Work out the finished part from the listing and answer in its coordinate system (mm). A direction names the side the tool comes from. Coordinates: 2 decimals unless noted, no trailing zeros. Order: outer loops, then holes, each group sorted by start corner. A loop starts at its lowest first (then second) coordinate and runs counter-clockwise, first axis right, second up.
```python
from build123d import *

# Parameters (mm, degrees)
SKETCH058_W          = 85
SKETCH058_H          = 10
SKETCH058_R          = 1.6
PAD030_DEPTH         = 10
FILLET019_R          = 3
SKETCH059_W          = 80
SKETCH059_H          = 5
PAD031_DEPTH         = 10
SKETCH060_W          = 61
SKETCH060_H          = 3.5
POCKET027_DEPTH      = 10.001
FILLET020_R          = 4
CHAMFER014_SIZE      = 5
SKETCH061_R          = 1.6
POCKET028_DEPTH      = 10.001
POCKET028_DEPTH_BACK = 5.001
CHAMFER015_SIZE      = 1.9
SKETCH062_R          = 2.3
POCKET029_DEPTH      = 7
CHAMFER016_SIZE      = 1
FILLET021_R          = 10
FILLET022_R          = 3
CHAMFER017_SIZE      = 0.5
SKETCH063_R          = 3.5
POCKET030_DEPTH      = 3
SKETCH064_R          = 3.5
POCKET031_DEPTH      = 3
SKETCH065_W          = 72
SKETCH065_H          = 3.5
POCKET032_DEPTH      = 10.001
FILLET023_R          = 2
FILLET024_R          = 5
CHAMFER018_SIZE      = 1
CHAMFER019_SIZE      = 1
CHAMFER020_SIZE      = 0.4


with BuildPart() as part:
    # Sketch058 → Pad030 (new body)
    with BuildSketch(Plane.XY):
        with Locations((-37.5, 0)):
            Rectangle(SKETCH058_W, SKETCH058_H)
        Circle(SKETCH058_R, mode=Mode.SUBTRACT)
    extrude(amount=PAD030_DEPTH)

    # Fillet019
    fillet019_edges = [part.edges().sort_by_distance(p)[0] for p in [
        (5, 5, 5),
        (5, -5, 5),
    ]]
    fillet(fillet019_edges, radius=FILLET019_R)

    # Sketch059 → Pad031 (join)
    with BuildSketch(Plane.XY):
        with Locations((-40, 7.5)):
            Rectangle(SKETCH059_W, SKETCH059_H)
    extrude(amount=PAD031_DEPTH)

    # Sketch060 → Pocket027 (cut, through all)
    with BuildSketch(Plane.XY):
        with Locations((-46.5, 6.25)):
            Rectangle(SKETCH060_W, SKETCH060_H)
    extrude(amount=POCKET027_DEPTH, mode=Mode.SUBTRACT)

    # Fillet020
    fillet020_edges = [part.edges().sort_by_distance(p)[0] for p in [
        (0, 10, 5),
        (-80, 10, 5),
    ]]
    fillet(fillet020_edges, radius=FILLET020_R)

    # Chamfer014
    chamfer014_edges = [part.edges().sort_by_distance(p)[0] for p in [
        (-80, -5, 5),
    ]]
    chamfer(chamfer014_edges, length=CHAMFER014_SIZE)

    # Sketch061 → Pocket028 (cut, two sides)
    with BuildSketch(Plane.XZ) as pocket028_sk:
        with Locations((-23, 5)):
            Circle(SKETCH061_R)
        with Locations((-70, 5)):
            Circle(SKETCH061_R)
    extrude(amount=-POCKET028_DEPTH, mode=Mode.SUBTRACT)
    extrude(pocket028_sk.sketch, amount=POCKET028_DEPTH_BACK, mode=Mode.SUBTRACT)

    # Chamfer015
    chamfer015_edges = [part.edges().sort_by_distance(p)[0] for p in [
        (-71.6, 10, 5),
        (-24.6, 10, 5),
    ]]
    chamfer(chamfer015_edges, length=CHAMFER015_SIZE)

    # Sketch062 (on Face11 of Chamfer015) → Pocket029 (cut)
    with BuildSketch(Plane.XZ.offset(5)):
        with Locations((-70, 5)):
            Circle(SKETCH062_R)
        with Locations((-23, 5)):
            Circle(SKETCH062_R)
    extrude(amount=-POCKET029_DEPTH, mode=Mode.SUBTRACT)

    # Chamfer016
    chamfer016_edges = [part.edges().sort_by_distance(p)[0] for p in [
        (-72.3, -5, 5),
        (-25.3, -5, 5),
    ]]
    chamfer(chamfer016_edges, length=CHAMFER016_SIZE)

    # Fillet021
    fillet021_edges = [part.edges().sort_by_distance(p)[0] for p in [
        (-80, 0, 5),
    ]]
    fillet(fillet021_edges, radius=FILLET021_R)

    # Fillet022
    fillet022_edges = [part.edges().sort_by_distance(p)[0] for p in [
        (-75, -5, 5),
    ]]
    fillet(fillet022_edges, radius=FILLET022_R)

    # Chamfer017
    chamfer017_edges = [part.edges().sort_by_distance(p)[0] for p in [
        (-71.6, 4.5, 5),
        (-24.6, 4.5, 5),
    ]]
    chamfer(chamfer017_edges, length=CHAMFER017_SIZE)

    # Sketch063 (on Face6 of Chamfer017) → Pocket030 (cut)
    with BuildSketch(Plane.XY.offset(10)):
        Circle(SKETCH063_R)
    extrude(amount=-POCKET030_DEPTH, mode=Mode.SUBTRACT)

    # Sketch064 (on Face3 of Pocket030) → Pocket031 (cut)
    with BuildSketch(Plane(origin=(0, 0, 0), x_dir=(1, 0, 0), z_dir=(0, 0, -1))):
        Circle(SKETCH064_R)
    extrude(amount=-POCKET031_DEPTH, mode=Mode.SUBTRACT)

    # Sketch065 → Pocket032 (cut, through all)
    with BuildSketch(Plane.XY):
        with Locations((-44, -3.25)):
            Rectangle(SKETCH065_W, SKETCH065_H)
    extrude(amount=POCKET032_DEPTH, mode=Mode.SUBTRACT)

    # Fillet023
    fillet023_edges = [part.edges().sort_by_distance(p)[0] for p in [
        (-8, -5, 5),
    ]]
    fillet(fillet023_edges, radius=FILLET023_R)

    # Fillet024
    fillet024_edges = [part.edges().sort_by_distance(p)[0] for p in [
        (-78.256289, -1.5, 5),
    ]]
    fillet(fillet024_edges, radius=FILLET024_R)

    # Chamfer018
    chamfer018_edges = [part.edges().sort_by_distance(p)[0] for p in [
        (-8, -1.5, 5),
    ]]
    chamfer(chamfer018_edges, length=CHAMFER018_SIZE)

    # Chamfer019
    chamfer019_edges = [part.edges().sort_by_distance(p)[0] for p in [
        (-72.3, -1.5, 5),
        (-25.3, -1.5, 5),
    ]]
    chamfer(chamfer019_edges, length=CHAMFER019_SIZE)

    # Chamfer020
    chamfer020_edges = [part.edges().sort_by_distance(p)[0] for p in [
        (-41.979297, -1.5, 10),
        (-8.5, -2, 10),
        (-78.259301, -0.255708, 10),
        (-8, -2.75, 10),
        (-79.979276, 3.498666, 10),
        (-7.414214, -4.414214, 10),
        (-80, 5.071068, 10),
        (-2, -5, 10),
        (-78.828427, 8.828427, 10),
        (4.12132, -4.12132, 10),
        (-40, 10, 10),
        (5, 0, 10),
        (-1.171573, 8.828427, 10),
        (4.12132, 4.12132, 10),
        (0, 5.5, 10),
        (1, 5, 10),
        (-3.5, 0, 10),
        (-46.5, 8, 10),
        (-16, 6.25, 10),
        (-77, 6.25, 10),
        (-46.5, 4.5, 10),
        (-41.979297, -1.5, 0),
        (-8.5, -2, 0),
        (-78.259301, -0.255708, 0),
        (-8, -2.75, 0),
        (-79.979276, 3.498666, 0),
        (-7.414214, -4.414214, 0),
        (-80, 5.071068, 0),
        (-2, -5, 0),
        (-78.828427, 8.828427, 0),
        (4.12132, -4.12132, 0),
        (-40, 10, 0),
        (5, 0, 0),
        (-1.171573, 8.828427, 0),
        (4.12132, 4.12132, 0),
        (0, 5.5, 0),
        (1, 5, 0),
        (-3.5, 0, 0),
        (-46.5, 8, 0),
        (-77, 6.25, 0),
        (-16, 6.25, 0),
        (-46.5, 4.5, 0),
    ]]
    chamfer(chamfer020_edges, length=CHAMFER020_SIZE)


solid = part.part
```
1. Flat-ended cylindrical pins translate along their axes: pin 1 (0.6 mm diameter, centred on y = -2.5, z = 3, fed in from -X); pin 2 (5 mm diameter, centred on x = -23, z = 5, fed in from -Y); pin 3 (1 mm diameter, centred on x = -48.5, z = 3, fed in from -Y). Find the tip coordinate at first contact, or state that the pin passes through.
2. The mould has two halves that part along Z. Classify faces 3 (the cylindrical face through (-22.26, 2.99, 3.58)), 4 (the cylindrical face through (-7.4, -4.43, 5.06)), 5 (the flat face through (-38, 3, 0)), 6 (the flat face through (-8.37, -1.85, 9.8)): released by +Z, released by -Z, zero draft, split by the parting line, or undercut.
3. The part is cut by section A-A (x = -70). Count the separate pieces of the cut face and the enclosed holes in it, plus the area to 3 significant figures.
4. The part is cut by section B-B (x = -32.5). Determine the outline of the cut face in (y, z), plus the area to 3 significant figures.
5. Consider probe 1 along Y at (x, z) = (-59.5, 9.25); probe 2 along X at (y, z) = (3.25, 3.75); probe 3 along X at (y, z) = (3.5, 6.25). Determine where each line is inside the solid, lowest interval first.
6. For faces 1 (the flat face through (-16, 6, 5)), 2 (the cylindrical face through (4.1, -4.14, 5.06)), determine the directions among +Z, -Z, +X, -X, +Y, -Y from which every point of the face is accessible in a straight line to the end or side of a thin tool.
Worked out:
1. pin 1: stops at x = -8.3
1. pin 2: stops at y = -0.7
1. pin 3: stops at y = -1.5
2. face 3: undercut
2. face 4: zero draft
2. face 5: released by -Z
2. face 6: released by +Z
3. separate pieces: 4
3. enclosed holes: 0
3. area: 44.0 mm2
4. outline: (-1.5, 0.4) - (-1.1, 0) - (4.1, 0) - (4.5, 0.4) - (4.5, 9.6) - (4.1, 10) - (-1.1, 10) - (-1.5, 9.6) - close; (8, 0.4) - (8.4, 0) - (9.6, 0) - (10, 0.4) - (10, 9.6) - (9.6, 10) - (8.4, 10) - (8, 9.6) - close
4. area: 79.4 mm2
5. probe 1: y = -1.5 to 4.5, 8 to 10
5. probe 2: x = -79.96 to -71, -69 to -24, -22 to 4.73
5. probe 3: x = -79.98 to -71, -69 to -24, -22 to 4.6
6. face 1: +Z, -Z
6. face 2: +Z, -Z, +X, -Y
